Input: part model. Units: mm. Frame: model coordinates. Face numbers are marked on the shaded views. A direction names the side the tool comes from. Coordinates: 2 decimals unless noted, no trailing zeros. Loops run counter-clockwise (first coordinate to the right, second up) from the corner with the lowest first, then second, coordinate; pieces in that order, holes last.
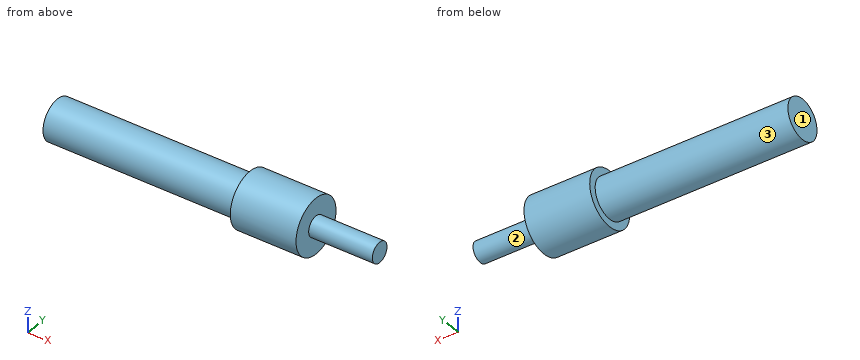
```python
from build123d import *

# Parameters (mm, degrees)
SKETCH1_R           = 6.48
BOSS_EXTRUDE1_DEPTH = 15.494
SKETCH2_R           = 4.715
BOSS_EXTRUDE2_DEPTH = 60.91
SKETCH3_R           = 2.375
BOSS_EXTRUDE3_DEPTH = 15


with BuildPart() as part:
    # Sketch1 → Boss-Extrude1 (new body)
    with BuildSketch(Plane.YZ):
        with Locations(Location((0, 0, 0), (0, 0, 270))):
            Circle(SKETCH1_R)
    extrude(amount=BOSS_EXTRUDE1_DEPTH)

    # Sketch2 → Boss-Extrude2 (add)
    with BuildSketch(Plane.YZ.offset(15.494)):
        with Locations(Location((0, 0, 0), (0, 0, 270))):
            Circle(SKETCH2_R)
    extrude(amount=-BOSS_EXTRUDE2_DEPTH)

    # Sketch3 → Boss-Extrude3 (add)
    with BuildSketch(Plane(origin=(15.494, 0, 0), x_dir=(0, -1, 0), z_dir=(-1, 0, 0))):
        with Locations(Location((0, 0, 0), (0, 0, 90))):
            Circle(SKETCH3_R)
    extrude(amount=-BOSS_EXTRUDE3_DEPTH)


solid = part.part
```
Item 1: Reachability of the marked faces 1, 2 and 3 from +Z, -Z, +X, -X, +Y, -Y: full face, straight path, thin tool, end or side. Return the list, or none.
Result:
face 1: +Z, -Z, -X, +Y, -Y
face 2: +X
face 3: -X
Item 2: Section query D-D (y = -3.25). Output: boundary loops of the cut face in (x, z).
Result:
outline: (-45.42, -3.42) - (0, -3.42) - (0, -5.61) - (15.49, -5.61) - (15.49, 5.61) - (0, 5.61) - (0, 3.42) - (-45.42, 3.42) - close
Item 3: Contact query for flat-ended pins moving along their axis: P1, Ø4, axis at y = -2.5, z = 2, coming from the +X side; P2, Ø2, axis at x = 15.5, z = -3.5, coming from the +Y side; P3, Ø6, axis at x = -10, z = -3, coming from the -Y side (3 decimals); P4, Ø1.5, axis at x = -12.5, y = 5, coming from the -Z side. Output: stop coordinate, or through.
Result:
P1: stops at x = 30.49
P2: stops at y = 5.98
P3: stops at y = -4.715
P4: stops at z = -2.04
Item 4: Section query C-C (x = -21). Output: boundary loops of the cut face in (y, z) (3 decimals).
Result:
outline: circle Ø9.43 at (0, 0)
Item 5: Line query: L1, parallel to X at y = -4.75, z = 2.75; L2, parallel to Y at x = -28, z = -0.25; L3, parallel to X at y = -4.25, z = 0.75. Output: solid intervals per line, ascending.
Result:
L1: x = 0 to 15.49
L2: y = -4.71 to 4.71
L3: x = -45.42 to 15.49
Item 6: Section query A-A (y = 0). Output: boundary loops of the cut face in (x, z) (3 decimals), then the cut area to 3 significant figures.
Result:
outline: (-45.416, -4.715) - (0, -4.715) - (0, -6.48) - (15.494, -6.48) - (15.494, -2.375) - (30.494, -2.375) - (30.494, 2.375) - (15.494, 2.375) - (15.494, 6.48) - (0, 6.48) - (0, 4.715) - (-45.416, 4.715) - close
area: 700 mm2
